Can you work these out from the model? Positions are in its coordinate system, mm. A direction names the side the tool comes from. Give positions to 0.01 mm unless a question says otherwise; leave off trailing zeros. Order: outer loops, then holes, each group sorted by start corner. A loop starts at its lowest first (then second) coordinate and runs counter-clockwise, first axis right, second up.
Item 1: If we mould it in two halves opening along X, with no side actions, what happens to faces 5 (the flat face through (-4.8, -11, 14)), 6 (the flat face through (-11, 1, 17.25)), 7 (the flat face through (7.5, -11, 14)), 8 (the flat face through (3, 2, 26))? For each: +X half, -X half, draft (parallel to the pull), parting line (faces both ways), or undercut.
Item 2: Which directions (+Z, -Z, +X, -X, +Y, -Y) give clear straight access to the entire face, cutting with the end or side of a thin tool? Please do faces 1 (the flat face through (-8.5, 8, 14)), 2 (the flat face through (3, 2, 2)), 3 (the flat face through (-11, -4.8, 14)), 4 (the flat face through (1, -11, 17.25)).
Item 3: I'm going to push flat-ended pins straight in: pin 1 Ø12 at (y, z) = (2, 6.5) entering from +X; pin 2 Ø6 at (y, z) = (6, 10) entering from +X; pin 3 Ø2 at (x, z) = (-0.5, 7) entering from +Y. Where does each tip first touch, or does it pass through?
Item 4: I want a section at A-A, the plane y = 0. Write out the boundary of the cut face in (x, z).
Item 5: I want a section at C-C, the plane z = 15. Write out the boundary of the cut face in (x, y).
Item 6: I want a section at B-B, the plane x = 3.25. Write out the boundary of the cut face in (y, z).
Item 7: I want a section at D-D, the plane x = -9. Write out the boundary of the cut face in (y, z), then the cut area to 3 significant figures.
Item 8: If I drill on line 1 along Z through (x, y) = (-10.5, 3.75); line 2 along Z through (x, y) = (8.5, -6.5); line 3 along X through (y, z) = (-9.75, 15), over which ranges is the centre line in solid material (lowest first)?
Autodesk Inventor part; units mm, degrees
ref_plane "Pracovní rovina3" through (13.5, -13.5, 0) normal (-1, 0, 0) x (0, 0, 1)
ref_plane "YZ Plane" through (0, 0, 0) normal (1, 0, 0) x (0, 1, 0)
ref_plane "XZ Plane" through (0, 0, 0) normal (0, 1, 0) x (-1, 0, 0)
sketch "Náčrt1" plane through (0, 0, 0) normal (0, 0, 1) x (1, 0, 0)
  line L0 (-18.9, 0) -> (18.9, 0)
  line L1 (0, 18.9) -> (0, -18.9)
  line L2 (-13.5, -13.5) -> (13.5, -13.5)
  line L3 (13.5, -13.5) -> (13.5, -8.5)
  line L4 (13.5, -8.5) -> (-8.5, 13.5)
  line L5 (-8.5, 13.5) -> (-13.5, 13.5)
  line L6 (-13.5, 13.5) -> (-13.5, -13.5)
  point P0 (0, 0)
  dimension "d0" = 27
  dimension "d1" = 27
  dimension "d2" = 5
  dimension "d3" = 5
extrude "Vysunutí1" add sketch "Náčrt1" along normal blind 28
ref_plane "Pracovní rovina3" through (13.5, -13.5, 0) normal (-1, 0, 0) x (0, 0, 1)
sketch "Náčrt5" plane through (13.5, -13.5, 0) normal (-1, 0, 0) x (0, 0, 1)
  line L0 (0, 5) -> (0, 27)
  line L1 (0, 27) -> (28, 27)
  line L2 (28, 5) -> (28, 27)
  line L3 (0, 5) -> (28, 5)
  line L4 (24, 27) -> (4, 27)
  line L5 (4, 27) -> (4, 5)
  line L6 (4, 5) -> (24, 5)
  line L7 (24, 5) -> (24, 27)
  point P0 (0, 13.5)
  dimension "d24" = 20
  dimension "d25" = 4
extrude "Vysunutí5" cut sketch "Náčrt5" along normal blind 22 contours L5 L1 L7 L3
sketch "Náčrt6" plane through (-13.5, -13.5, 0) normal (-1, 0, 0) x (0, 0, 1)
  line L0 (0, 27) -> (0, 0)
  line L1 (0, 0) -> (28, 0)
  line L2 (28, 27) -> (28, 0)
  line L3 (0, 27) -> (28, 27)
  line L4 (10.75, 21) -> (17.25, 21)
  line L5 (17.25, 21) -> (17.25, 8.7)
  line L6 (17.25, 8.7) -> (10.75, 8.7)
  line L7 (10.75, 8.7) -> (10.75, 21)
  point P0 (0, 13.5)
  dimension "d28" = 6.5
  dimension "d29" = 12.3
  dimension "d30" = 10.75
  dimension "d31" = 6
extrude "Vysunutí6" cut sketch "Náčrt6" against normal through all contours L4 L5 L6 L7
pattern_circular "Kruhové pole1" count 2 over 90 about axis through (-13.5, -13.5, 0) along (0, 0, -1) of "Vysunutí6"
sketch "Náčrt7" plane through (-13.5, -13.5, 0) normal (0, -1, 0) x (1, 0, 0)
  line L0 (0, 0) -> (27, 0)
  line L1 (27, 0) -> (27, 28)
  line L2 (0, 28) -> (27, 28)
  line L3 (0, 0) -> (0, 28)
  line L4 (-5.4, 0) -> (32.4, 0)
  line L5 (-5.4, 0) -> (32.4, 0)
  line L6 (13.5, -5.6) -> (13.5, 33.6)
  line L7 (21, 17.25) -> (8.7, 17.25)
  line L8 (8.7, 17.25) -> (8.7, 10.75)
  line L9 (8.7, 10.75) -> (21, 10.75)
  line L10 (21, 10.75) -> (21, 17.25)
  point P0 (13.5, 0)
  dimension "d37" = 12.3
  dimension "d38" = 6.5
  dimension "d39" = 6
  dimension "d40" = 10.75
extrude "Vysunutí7" cut sketch "Náčrt7" against normal through all contours L9 L8 L7 L6 | L6 L7 L10 L9
properties part number "masterpiece_uhelnik_3D tisk"
Results list:
1. face 5: undercut
1. face 6: draft
1. face 7: undercut
1. face 8: +X half
2. face 1: +X, +Y
2. face 2: +Z, -Z, +X, +Y
2. face 3: +X, -X
2. face 4: +Y, -Y
3. pin 1: stops at x = 8.45
3. pin 2: stops at x = -8.5
3. pin 3: stops at y = -8.5
4. outline: (-13.5, 0) - (5, 0) - (5, 4) - (-8.5, 4) - (-8.5, 10.75) - (-13.5, 10.75) - close; (-13.5, 17.25) - (-8.5, 17.25) - (-8.5, 24) - (5, 24) - (5, 28) - (-13.5, 28) - close
5. outline: (-13.5, -13.5) - (-4.8, -13.5) - (-4.8, -8.5) - (-8.5, -8.5) - (-8.5, -4.8) - (-13.5, -4.8) - close; (-13.5, 7.5) - (-8.5, 7.5) - (-8.5, 13.5) - (-13.5, 13.5) - close; (7.5, -13.5) - (13.5, -13.5) - (13.5, -8.5) - (7.5, -8.5) - close
6. outline: (-13.5, 0) - (1.75, 0) - (1.75, 4) - (-8.5, 4) - (-8.5, 10.75) - (-13.5, 10.75) - close; (-13.5, 17.25) - (-8.5, 17.25) - (-8.5, 24) - (1.75, 24) - (1.75, 28) - (-13.5, 28) - close
7. outline: (-13.5, 0) - (13.5, 0) - (13.5, 28) - (-13.5, 28) - close; hole (-4.8, 10.75) - (7.5, 10.75) - (7.5, 17.25) - (-4.8, 17.25) - close
7. area: 676 mm2
8. line 1: z = 0 to 10.75, 17.25 to 28
8. line 2: z = 0 to 4, 24 to 28
8. line 3: x = -13.5 to -4.8, 7.5 to 13.5
